from build123d import *

# Parameters (mm, degrees)
BOSS_EXTRUDE1_DEPTH = 25
SKETCH2_R           = 14.285
CUT_EXTRUDE1_DEPTH  = 487.882938036


with BuildPart() as part:
    # Sketch1 → Boss-Extrude1 (new body)
    with BuildSketch(Plane.XY):
        with BuildLine():
            Line((0, 470), (102.304530941, 470))
            ThreePointArc((102.304530941, 470), (115.701411141, 464.850037068), (122.198947697, 452.052360092))
            add(Edge.make_bspline(
                [(122.198947697, 452.052360092), (126.05707976, 414.653812215), (124.54872054, 341.079870989), (104.591114629, 269.95223882), (90, 235)],
                knots=[0.073881588, 0.073881588, 0.073881588, 0.073881588, 0.536940794, 1, 1, 1, 1], degree=3))
            add(Edge.make_bspline(
                [(90, 235), (98.310393886, 211.902473229), (109.325776263, 152.77450372), (109.130347847, 67.78070228), (106.22993094, 18.817343576)],
                knots=[0, 0, 0, 0, 0.470365123, 0.940730246, 0.940730246, 0.940730246, 0.940730246], degree=3))
            ThreePointArc((106.22993094, 18.817343576), (99.982560761, 5.445737249), (86.264928467, 0))
            Line((86.264928467, 0), (0, 0))
            Line((0, 0), (-86.264928467, 0))
            ThreePointArc((-86.264928467, 0), (-99.982560761, 5.445737249), (-106.22993094, 18.817343576))
            add(Edge.make_bspline(
                [(-90, 235), (-98.310393886, 211.902473229), (-109.325776263, 152.77450372), (-109.130347847, 67.78070228), (-106.22993094, 18.817343576)],
                knots=[0, 0, 0, 0, 0.470365123, 0.940730246, 0.940730246, 0.940730246, 0.940730246], degree=3))
            add(Edge.make_bspline(
                [(-122.198947697, 452.052360092), (-126.05707976, 414.653812215), (-124.54872054, 341.079870989), (-104.591114629, 269.95223882), (-90, 235)],
                knots=[0.073881588, 0.073881588, 0.073881588, 0.073881588, 0.536940794, 1, 1, 1, 1], degree=3))
            ThreePointArc((-122.198947697, 452.052360092), (-115.701411141, 464.850037068), (-102.304530941, 470))
            Line((-102.304530941, 470), (0, 470))
        make_face()
    extrude(amount=BOSS_EXTRUDE1_DEPTH)

    # Sketch2 → Cut-Extrude1 (cut, through all)
    with BuildSketch(Plane(origin=(0, 0, 0), x_dir=(1, 0, 0), z_dir=(0, 1, 0))):
        Circle(SKETCH2_R)
    extrude(amount=CUT_EXTRUDE1_DEPTH, mode=Mode.SUBTRACT)


solid = part.part
Build history of the part. All positions in model axes, mm. Coordinates: 2 decimals unless noted, no trailing zeros. Order: outer loops, then holes, each group sorted by start corner. A loop starts at its lowest first (then second) coordinate and runs counter-clockwise, first axis right, second up. Notation, with made-up numbers: (15, 73.5) -> (30, 73.5) arc R14 cw to (30, 79.5) -> close; hole circle Ø7 at (6, 45.5). An arc over 180 degrees is marked (long way). One line per item, written item: value.
(1) Slice it at A-A, the plane x = 0. List the corners of the cut face in (y, z) (3 decimals), plus the area to 3 significant figures.
Checked values:
outline: (0, 14.285) -> (470, 14.285) -> (470, 25) -> (0, 25) -> close
area: 5,040 mm2
(2) Drop a flat-ended pin along its axis: pin 1 Ø3 at (y, z) = (206, 20.5) entering from -X. Give the stop position or say it passes through.
Checked values:
pin 1: x = -98.56
(3) Probe line 1 (X direction, y = 48.5, z = 1.75); line 2 (X direction, y = 44.5, z = 3.75); line 3 (X direction, y = 284, z = 22.75). List the from-to ranges inside material, lowest first. Write a range as [from, to].
Checked values:
line 1: [-107.67, -14.18], [14.18, 107.67]
line 2: [-107.52, -13.78], [13.78, 107.52]
line 3: [-107.32, 107.32]
(4) Mould opens along X. For faces 1 (the cylindrical face through (-115.853, 464.712, 12.325)), 2 (the flat face through (59, 238, 0)), 3 (the cylindrical face through (-0.31, 231.71, 14.28)), 4 (the cylindrical face through (115.548, 464.987, 12.325)) say: pulls with the +X half, pulls with the -X half, needs draft (parallel to the pull), parting line crosses it, or undercut.
Checked values:
face 1: pulls with the -X half
face 2: needs draft
face 3: undercut
face 4: pulls with the +X half
